from build123d import *

# Parameters (mm, degrees)
F0_W     = 137.16
F0_H     = 35.56
F1_DEPTH = 12.7
F2_R     = 10.1577407599
F3_DEPTH = 10.795
F4_R     = 3.15
F5_DEPTH = 1.905
F6_W     = 22.86
F6_H     = 1.27
F6_H_2   = 5.08
F6_W_2   = 1.27
F7_DEPTH = 50.8


with BuildPart() as f1:
    # F0 (on Top) → F1 (new body)
    with BuildSketch(Plane.XY):
        Rectangle(F0_W, F0_H)
    extrude(amount=F1_DEPTH)

    # F2 (on face) → F3 (cut)
    with BuildSketch(Plane(origin=(0, 0, 0), x_dir=(1, 0, 0), z_dir=(0, 0, -1))):
        with Locations((5.08, 0)):
            Circle(F2_R)
    extrude(amount=-F3_DEPTH, mode=Mode.SUBTRACT)

    # F4 (on face) → F5 (cut)
    with BuildSketch(Plane(origin=(0, 0, 10.795), x_dir=(1, 0, 0), z_dir=(0, 0, -1))):
        with Locations((5.08, 0)):
            Circle(F4_R)
    extrude(amount=-F5_DEPTH, mode=Mode.SUBTRACT)

    # F6 (on face) → F7 (cut)
    with BuildSketch(Plane.XZ.offset(17.78)):
        with Locations((55.88, 3.175)):
            Rectangle(F6_W, F6_H)
        with Locations((55.88, 6.35)):
            Rectangle(F6_W, F6_H_2)
        with Locations((43.815, 6.35)):
            Rectangle(F6_W_2, F6_H_2)
        with Locations((55.88, 9.525)):
            Rectangle(F6_W, F6_H)
        with Locations((67.945, 6.35)):
            Rectangle(F6_W_2, F6_H_2)
        with Locations((-55.88, 3.175)):
            Rectangle(F6_W, F6_H)
        with Locations((-55.88, 6.35)):
            Rectangle(F6_W, F6_H_2)
        with Locations((-67.945, 6.35)):
            Rectangle(F6_W_2, F6_H_2)
        with Locations((-43.815, 6.35)):
            Rectangle(F6_W_2, F6_H_2)
        with Locations((-55.88, 9.525)):
            Rectangle(F6_W, F6_H)
    extrude(amount=-F7_DEPTH, mode=Mode.SUBTRACT)


solid = f1.part
Geometry check sheet. Reference: the model listing, model coordinates, mm. A direction names the side the tool comes from. Round coordinates to 2 decimals unless told otherwise and drop trailing zeros. Loops run counter-clockwise (first coordinate to the right, second up) from the corner with the lowest first, then second, coordinate; pieces in that order, holes last. Notation, with made-up numbers: (3.5, 40) - (39.5, 40) arc R15 cw to (39.5, 62) - close; hole circle Ø6 at (39, -26.5). An arc over 180 degrees is marked (long way). One line per question, with ' | ' between items. Start each with the question number.
1. Draft check along Z on faces 4 (the face through (68.58, 0, 11)), 5 (the face through (-56, 0, 2.54)), 6 (the face through (2.7, -2.4, 10.795)), 7 (the face through (56, 0, 10.16)). Enter one of: released by +Z, released by -Z, zero draft, split by the parting line, or undercut.
2. Tool access check on faces 1 (the face through (-43.18, 0, 6)), 2 (the face through (56, 0, 2.54)), 3 (the face through (43.18, 0, 6)). Record the directions out of +Z, -Z, +X, -X, +Y, -Y that give a thin tool (end or side, any length) a straight path to the whole face; none if there is none.
3. Cross-section at A-A on x = 5.08. Record the cut outline in (y, z) (3 decimals).
4. Cross-section at B-B on y = -12. Record the cut outline in (x, z), then the cut area to 3 significant figures.
5. Cross-section at C-C on z = 6.5. Record the cut outline in (x, y), then the cut area to 3 significant figures.
6. Depth check by flat-ended pin: pin 1 (2.5 mm diameter, centred on y = 5.5, z = 5.5, fed in from +X); pin 2 (6 mm diameter, centred on x = 1.5, y = 1, fed in from -Z) (3 decimals). Enter the tip coordinate at first touch or a pass-through.
7. Scan lines: line 1 (X direction, y = 0, z = 3.5); line 2 (X direction, y = -16, z = 9); line 3 (Y direction, x = 5.08, z = 11.7). Record each from-to range of solid material in increasing order. Write a range as [from, to].
Taken from the geometry:
1) face 4: zero draft | face 5: undercut | face 6: released by -Z | face 7: undercut
2) face 1: -X, +Y, -Y | face 2: +Y, -Y | face 3: +X, +Y, -Y
3) outline: (-17.78, 0) - (-10.158, 0) - (-10.158, 10.795) - (-3.15, 10.795) - (-3.15, 12.7) - (-17.78, 12.7) - close; (3.15, 10.795) - (10.158, 10.795) - (10.158, 0) - (17.78, 0) - (17.78, 12.7) - (3.15, 12.7) - close
4) outline: (-68.58, 0) - (68.58, 0) - (68.58, 3.81) - (67.31, 3.81) - (67.31, 2.54) - (44.45, 2.54) - (44.45, 3.81) - (43.18, 3.81) - (43.18, 8.89) - (44.45, 8.89) - (44.45, 10.16) - (67.31, 10.16) - (67.31, 8.89) - (68.58, 8.89) - (68.58, 12.7) - (-68.58, 12.7) - (-68.58, 8.89) - (-67.31, 8.89) - (-67.31, 10.16) - (-44.45, 10.16) - (-44.45, 8.89) - (-43.18, 8.89) - (-43.18, 3.81) - (-44.45, 3.81) - (-44.45, 2.54) - (-67.31, 2.54) - (-67.31, 3.81) - (-68.58, 3.81) - close | area: 1,370 mm²
5) outline: (-43.18, -17.78) - (43.18, -17.78) - (43.18, 17.78) - (-43.18, 17.78) - close; hole circle Ø20.32 at (5.08, 0) | area: 2,750 mm²
6) pin 1: x = 43.18 | pin 2: z = 10.795
7) line 1: [-68.58, -67.31], [-44.45, -5.08], [15.24, 44.45], [67.31, 68.58] | line 2: [-68.58, -67.31], [-44.45, 44.45], [67.31, 68.58] | line 3: [-17.78, -3.15], [3.15, 17.78]
